Geometry check sheet. Reference: the model listing, model coordinates, mm. A direction names the side the tool comes from. Coordinates: 2 decimals unless noted, no trailing zeros. Loops run counter-clockwise (first coordinate to the right, second up) from the corner with the lowest first, then second, coordinate; pieces in that order, holes last. Notation, with made-up numbers: (16, -31) - (65, -31) arc R27 cw to (65, -6) - close; hole circle Ø5 at (23, -25.5). An arc over 180 degrees is marked (long way). One line per item, written item: value.
from build123d import *

# Parameters (mm, degrees)
EXTRUDE_4_DEPTH = 80


with BuildPart() as part:
    # 草圖1 → 填料-伸長4 (new body)
    with BuildSketch(Plane.XY):
        Polygon((-0.045443236, -0.270925117), (-10.045443236, -0.270925117), (-35.045443236, -0.270925117), (-35.045443236, -5.270925117), (34.954556764, -5.270925117), (34.954556764, -0.270925117), align=None)
        Polygon((2.843781018, 49.729074883), (-10.045443236, -0.270925117), (-0.045443236, -0.270925117), (12.843781018, 49.729074883), align=None)
        Polygon((-35.045443236, -0.270925117), (-10.045443236, -0.270925117), (-28.827398823, 4.355440349), (-26.239696609, 14.22289864), (-31.239662656, 14.241324755), align=None)
    extrude(amount=EXTRUDE_4_DEPTH)


solid = part.part
(1) Cross-section at C-C on x = 25. Record the cut outline in (y, z).
Reply:
outline: (-5.27, 0) - (-0.27, 0) - (-0.27, 80) - (-5.27, 80) - close
(2) Cross-section at B-B on z = 62.5. Record the cut outline in (x, y), and give its area (3 significant figures).
Reply:
outline: (-35.05, -5.27) - (34.95, -5.27) - (34.95, -0.27) - (-0.05, -0.27) - (12.84, 49.73) - (2.84, 49.73) - (-10.05, -0.27) - (-28.83, 4.36) - (-26.24, 14.22) - (-31.24, 14.24) - (-35.05, -0.27) - close
area: 969 mm2
(3) Release check for a two-part mould opening along X. For faces 1 (the face through (-33.116, 7.087, 39.44)), 2 (the face through (-19.3, 2.01, 39.44)), 3 (the face through (34.955, -3, 39)) record: pulls with the +X half, pulls with the -X half, needs draft (parallel to the pull), parting line crosses it, or undercut.
Reply:
face 1: pulls with the -X half
face 2: undercut
face 3: pulls with the +X half
(4) Access from +Z, -Z, +X, -X, +Y, -Y to the whole of each face (thin tool, end or side, straight path). Record for faces 4 (the face through (18, -0.271, 39)), 5 (the face through (-3, 12, 80)), 6 (the face through (-27.55, 9.22, 39.44)), 7 (the face through (8, 49.729, 39)), 8 (the face through (-3.51, 25.08, 39.44)).
Reply:
face 4: +Z, -Z, +X
face 5: +Z, +X, -X, +Y, -Y
face 6: +Z, -Z
face 7: +Z, -Z, +X, -X, +Y
face 8: +Z, -Z, +Y
(5) Material ranges on probe 1 along Y at (x, z) = (18, 73.5); probe 2 along X at (y, z) = (12, 11); probe 3 along X at (y, z) = (25, 21), recorded low to high. Write a range as from..to.
Reply:
probe 1: -5.27..-0.27
probe 2: -31.83..-26.82, -6.88..3.12
probe 3: -3.53..6.47
(6) Go/stop test with flat-tipped pins: pin 1 Ø8 at (y, z) = (15.5, 46) entering from +X; pin 2 Ø1 at (x, y) = (-24.5, 5.5) entering from +Z; pin 3 Ø3 at (y, z) = (7, 35.5) entering from +X; pin 4 Ø6 at (y, z) = (20, 51.5) entering from -X. Record where each tip stops, or that it passes through.
Reply:
pin 1: x = 5.05
pin 2: through
pin 3: x = 2.22
pin 4: x = -5.59
(7) Cross-section at A-A on y = 11.5. Record the cut outline in (x, z), and give its area (3 significant figures).
Reply:
outline: (-31.96, 0) - (-26.95, 0) - (-26.95, 80) - (-31.96, 80) - close; (-7.01, 0) - (2.99, 0) - (2.99, 80) - (-7.01, 80) - close
area: 1,200 mm2
(8) Cross-section at D-D on y = 26. Record the cut outline in (x, z).
Reply:
outline: (-3.27, 0) - (6.73, 0) - (6.73, 80) - (-3.27, 80) - close
